Input: dimensioned drawing with shaded views. Units: mm. Origin: part minimum x, y, z. A direction names the side the tool comes from. Give positions to 0.01 mm unless a question says otherwise; leave off trailing zeros. Loops run counter-clockwise (first coordinate to the right, second up) from the corner with the lowest first, then second, coordinate; pieces in that order, holes last.
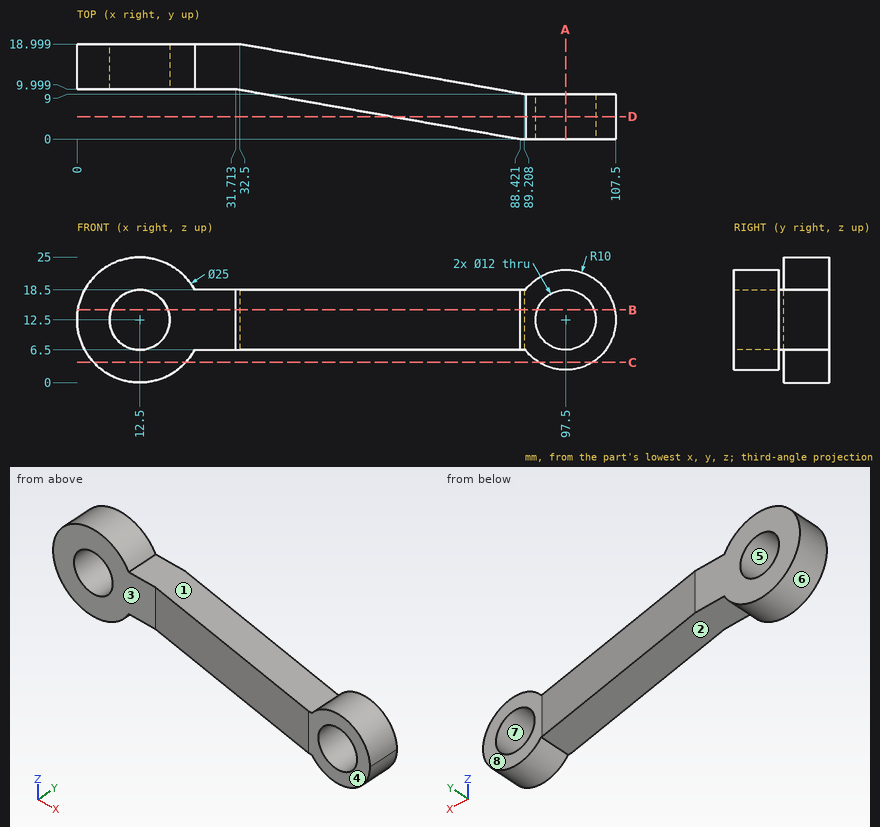
(1) Section C-C, the plane z = 4. Return the cut outline in (x, y) (1 decimal).
A:
outline: (3.3, 10) - (21.7, 10) - (21.7, 19) - (3.3, 19) - close; (92.2, 0) - (102.8, 0) - (102.8, 9) - (92.2, 9) - close
(2) Section D-D, the plane y = 4.5. Return the cut outline in (x, z), then the cut area to 3 significant figures.
A:
outline: (62.9, 6.5) - (89.5, 6.5) arc R10 ccw (long way) to (89.5, 18.5) - (62.9, 18.5) - close; hole circle Ø12 at (97.5, 12.5)
area: 504 mm2
(3) First-contact query: pin 1 (14 mm diameter, centred on x = 12.5, z = 12.5, fed in from -Y); pin 2 (1.5 mm diameter, centred on x = 75.5, z = 17, fed in from -Y); pin 3 (3 mm diameter, centred on x = 24, y = 14.5, fed in from +Z). Flat tips, straight axial feed; report the tip coordinate or a pass-through.
A:
pin 1: stops at y = 10
pin 2: stops at y = 2.15
pin 3: stops at z = 20
(4) Section B-B, the plane z = 14.5. Return the cut outline in (x, y).
A:
outline: (0.16, 10) - (6.84, 10) - (6.84, 19) - (0.16, 19) - close; (18.16, 10) - (31.71, 10) - (88.42, 0) - (91.84, 0) - (91.84, 9) - (89.21, 9) - (32.5, 19) - (18.16, 19) - close; (103.16, 0) - (107.3, 0) - (107.3, 9) - (103.16, 9) - close
(5) Mould query, pull axis Z, two halves, no side actions, for the marked faces 6, 7 and 8. Classes: pulls with the +Z half, pulls with the -Z half, needs draft (parallel to the pull), parting line crosses it, or undercut.
A:
face 6: parting line crosses it
face 7: undercut
face 8: needs draft
(6) Ray query, line 1 along Z through (x, y) = (13, 10.5); line 2 along Z through (x, y) = (97.5, 4); line 3 along Z through (x, y) = (82, 8.5). Return the intervals inside material, ascending.
A:
line 1: z = 0.01 to 6.52, 18.48 to 24.99
line 2: z = 2.5 to 6.5, 18.5 to 22.5
line 3: z = 6.5 to 18.5
(7) Reachability of the marked faces 1, 2, 3, 4 and 5 from +Z, -Z, +X, -X, +Y, -Y: full face, straight path, thin tool, end or side. Return the list, or none.
A:
face 1: +Z, +Y, -Y
face 2: -Z, +Y, -Y
face 3: +Z, -Z, -X, -Y
face 4: +Z, -Z, +X, -X, -Y
face 5: +Y, -Y
(8) Section A-A, the plane x = 97.5. Return the cut outline in (y, z).
A:
outline: (0, 2.5) - (9, 2.5) - (9, 6.5) - (0, 6.5) - close; (0, 18.5) - (9, 18.5) - (9, 22.5) - (0, 22.5) - close
